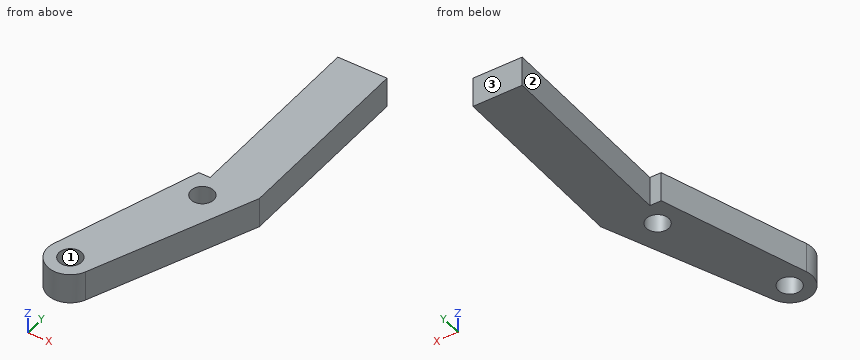
```python
from build123d import *

# Parameters (mm, degrees)
SKETCH1_R           = 1.499999946
SKETCH1_R_2         = 1.500000009
BOSS_EXTRUDE2_DEPTH = 4


# Read off the part's stored shape, not the designer's step: Imported1
with BuildPart() as part:
    # Sketch1 → Boss-Extrude2 (new body)
    with BuildSketch(Plane.XY.offset(4.00000019)):
        with BuildLine():
            Line((8.00000038, 47.970000654), (14.499999583, 47.970000654))
            Line((14.499999583, 47.970000654), (14.499999583, 22.970002145))
            Line((14.499999583, 22.970002145), (5.772520595, 1.854081769))
            ThreePointArc((5.772520595, 1.854081769), (1.951680977, 0.189123339), (0.154201944, 3.949438629))
            Line((0.154201944, 3.949438629), (6.500000134, 22.970002145))
            Line((6.500000134, 22.970002145), (8.00000038, 22.970002145))
            Line((8.00000038, 22.970002145), (8.00000038, 47.970000654))
        make_face()
        with Locations((9.000000172, 19.969999637)):
            Circle(SKETCH1_R, mode=Mode.SUBTRACT)
        with Locations((3.000000037, 2.99999995)):
            Circle(SKETCH1_R_2, mode=Mode.SUBTRACT)
    extrude(amount=BOSS_EXTRUDE2_DEPTH)


solid = part.part
```
Source: CAD feature listing. Evaluate the final solid. Frame: model axes, mm. Face numbers are marked on the shaded views. Round coordinates to 2 decimals unless told otherwise and drop trailing zeros. Loops run counter-clockwise (first coordinate to the right, second up) from the corner with the lowest first, then second, coordinate; pieces in that order, holes last. Notation, with made-up numbers: M 55.25,85 L 60.25,85 A17 cw 60.25,92 Z; hole C 84.5,85.5 d2. An arc over 180 degrees is marked long. Use a Markdown table: item, result. Add a question column.
1. Section query A-A on z = 7.1. Return the cut outline in (x, y).
2. Section query B-B on y = 3. Return the cut outline in (x, z), then the cut area to 3 significant figures.
3. Section query C-C on x = 4. Return the cut outline in (y, z), then the cut area to 3 significant figures.
4. Section query D-D on y = 40. Return the cut outline in (x, z).
5. Mould query, pull axis X, two halves, no side actions, for the marked faces 1, 2 and 3. Classes: pulls with the +X half, pulls with the -X half, needs draft (parallel to the pull), parting line crosses it, or undercut.
6. Contact query for flat-ended pins moving along their axis: P1, Ø1.5, axis at x = 9, z = 6, coming from the -Y side; P2, Ø1.2, axis at y = 36, z = 5.5, coming from the -X side; P3, Ø1.2, axis at x = 7, z = 5, coming from the +Y side; P4, Ø2.5, axis at x = 3, y = 3, coming from the +Z side. Output: stop coordinate, or through.
7. Line query: line 1 (X direction, y = 38, z = 7.15); line 2 (Y direction, x = 9, z = 4.85); line 3 (X direction, y = 3, z = 5.4). Output: solid intervals per line, ascending.
Reported:
| question | item | result |
|---|---|---|
| 1 | outline | M 0.15,3.95 A3 ccw 5.77,1.85 L 14.5,22.97 L 14.5,47.97 L 8,47.97 L 8,22.97 L 6.5,22.97 Z; hole C 3,3 d3; hole C 9,19.97 d3 |
| 2 | outline | M 0,4 L 1.5,4 L 1.5,8 L 0,8 Z; M 4.5,4 L 6.25,4 L 6.25,8 L 4.5,8 Z |
| 2 | area | 13.0 mm² |
| 3 | outline | M 0.17,4 L 1.88,4 L 1.88,8 L 0.17,8 Z; M 4.12,4 L 15.48,4 L 15.48,8 L 4.12,8 Z |
| 3 | area | 52.3 mm² |
| 4 | outline | M 8,4 L 14.5,4 L 14.5,8 L 8,8 Z |
| 5 | face 1 | undercut |
| 5 | face 2 | pulls with the -X half |
| 5 | face 3 | needs draft |
| 6 | P1 | stops at y = 7.85 |
| 6 | P2 | stops at x = 8 |
| 6 | P3 | stops at y = 22.97 |
| 6 | P4 | passes through |
| 7 | line 1 | x = 8 to 14.5 |
| 7 | line 2 | y = 9.66 to 18.47, 21.47 to 47.97 |
| 7 | line 3 | x = 0 to 1.5, 4.5 to 6.25 |
